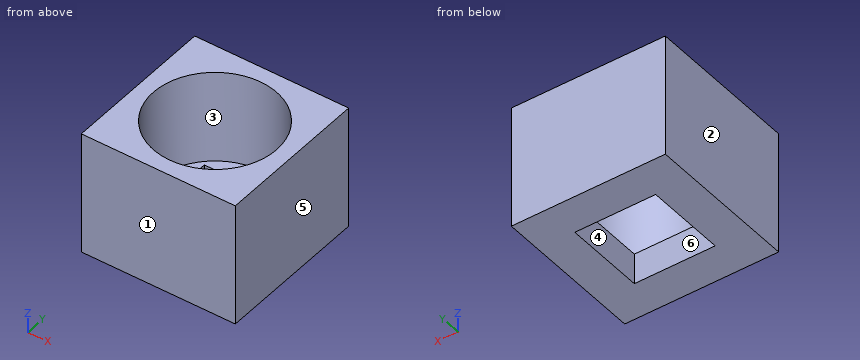
```python
from build123d import *

# Parameters (mm, degrees)
F0_W     = 10
F0_H     = 10
F1_DEPTH = 8
F2_R     = 4
F3_DEPTH = 6
F4_W     = 5.25
F4_H     = 5.25
F5_DEPTH = 3


# Not quite as in the source:
# - a feature names something its author has since deleted; it is built from what else it names


with BuildPart() as f1:
    # F0 (on Top) → F1 (new body)
    with BuildSketch(Plane.XY):
        Rectangle(F0_W, F0_H)
    extrude(amount=F1_DEPTH)

    # F2 (on face) → F3 (cut)
    with BuildSketch(Plane.XY.offset(8)):
        Circle(F2_R)
    extrude(amount=-F3_DEPTH, mode=Mode.SUBTRACT)

    # F4 (on face) → F5 (cut)
    with BuildSketch(Plane.XY):
        Rectangle(F4_W, F4_H)
    extrude(amount=F5_DEPTH, mode=Mode.SUBTRACT)


solid = f1.part
```
The listing builds one solid part. Answer for the finished solid, in the listing's coordinates (mm). Face numbers are marked on the shaded views. A direction names the side the tool comes from. Give positions to 0.01 mm unless a question says otherwise; leave off trailing zeros. Order: outer loops, then holes, each group sorted by start corner. A loop starts at its lowest first (then second) coordinate and runs counter-clockwise, first axis right, second up. Notation, with made-up numbers: (9, 85.25) - (29, 85.25) arc R16 ccw to (29, 92.25) - close; hole circle Ø10 at (-37.5, 74). An arc over 180 degrees is marked (long way). Use one line per item in the form item = value. Start each with the question number.
(1) A cutting plane is placed at D-D, the plane y = 3.75. Write down the section's boundary in (x, z).
(2) For the marked faces 5 and 6, determine the directions among +Z, -Z, +X, -X, +Y, -Y from which every point of the face is accessible in a straight line to the end or side of a thin tool.
(3) The mould has two halves that part along Y. Classify the marked faces 1, 2, 3 and 4: released by +Y, released by -Y, zero draft, split by the parting line, or undercut.
(4) Consider line 1 (X direction, y = -1.25, z = 0.75) (3 decimals); line 2 (Y direction, x = 0, z = 5.35); line 3 (Y direction, x = 2.75, z = 6). Determine where each line is inside the solid, lowest interval first. Write a range as from..to.
(5) A cutting plane is placed at A-A, the plane x = 0. Write down the section's boundary in (y, z) (3 decimals), then the cut area to 3 significant figures.
(6) A cutting plane is placed at C-C, the plane z = 1. Write down the section's boundary in (x, y) (3 decimals), then the cut area to 3 significant figures.
Ans:
q1.outline = (-5, 0) - (5, 0) - (5, 8) - (1.39, 8) - (1.39, 2) - (-1.39, 2) - (-1.39, 8) - (-5, 8) - close
q2.face_5 = +Z, -Z, +X, +Y, -Y
q2.face_6 = +Z, -Z
q3.face_1 = released by -Y
q3.face_2 = zero draft
q3.face_3 = undercut
q3.face_4 = undercut
q4.line_1 = -5..-2.625, 2.625..5
q4.line_2 = -5..-4, 4..5
q4.line_3 = -5..-2.9, 2.9..5
q5.outline = (-5, 0) - (-2.625, 0) - (-2.625, 2) - (-4, 2) - (-4, 8) - (-5, 8) - close; (2.625, 0) - (5, 0) - (5, 8) - (4, 8) - (4, 2) - (2.625, 2) - close
q5.area = 21.5 mm^2
q6.outline = (-5, -5) - (5, -5) - (5, 5) - (-5, 5) - close; hole (-2.625, -2.625) - (2.625, -2.625) - (2.625, 2.625) - (-2.625, 2.625) - close
q6.area = 72.4 mm^2
